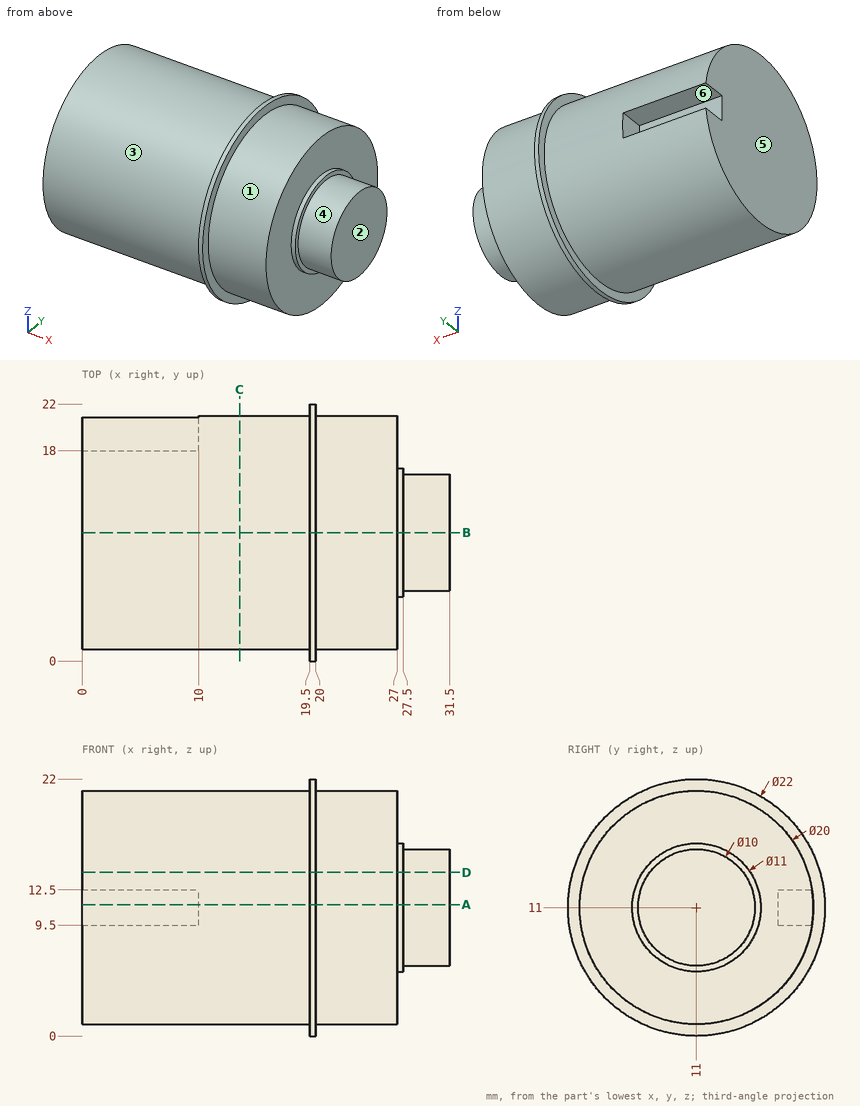
The drawing under review shows one solid part. Ordinate dimensions are in mm from its lowest x, y, z. A direction names the side the tool comes from. Round coordinates to 2 decimals unless told otherwise and drop trailing zeros. Order: outer loops, then holes, each group sorted by start corner. A loop starts at its lowest first (then second) coordinate and runs counter-clockwise, first axis right, second up. Notation, with made-up numbers: (7.25, 78.25) -> (64.25, 78.25) arc R17 cw to (64.25, 96.25) -> close; hole circle Ø5 at (65, 40.25). An arc over 180 degrees is marked (long way). Use a Markdown table: item, result.
Q1. We need section C-C on x = 13.5. Write out the cut boundary in (y, z), then the cut area to 3 significant figures.
Values:
| item | result |
|---|---|
| outline | circle Ø20 at (11, 11) |
| area | 314 mm^2 |
Q2. Clearance check with flat-ended pins moving along their axes: P1, Ø1.5, axis at y = 17.5, z = 11, coming from the +X side; P2, Ø3, axis at x = 6, y = 19.5, coming from the +Z side; P3, Ø2.5, axis at x = 6.5, y = 19.5, coming from the -Z side; P4, Ø6.5, axis at y = 12.5, z = 12.5, coming from the -X side. State where each tip first meets the part, or that it passes through.
Values:
| item | result |
|---|---|
| P1 | stops at x = 27 |
| P2 | stops at z = 18.14 |
| P3 | stops at z = 4.11 |
| P4 | stops at x = 0 |
Q3. For line 1 (X direction, y = 17.25, z = 15.25); line 2 (X direction, y = 4, z = 18.25); line 3 (Y direction, x = 29.5, z = 11.25), list the stretches that pass through material, from the lowest coordinate up.
Values:
| item | result |
|---|---|
| line 1 | x = 0 to 27 |
| line 2 | x = 19.5 to 20 |
| line 3 | y = 6.01 to 15.99 |
Q4. We need section D-D on z = 14. Write out the cut boundary in (x, y), then the cut area to 3 significant figures.
Values:
| item | result |
|---|---|
| outline | (0, 1.46) -> (19.5, 1.46) -> (19.5, 0.42) -> (20, 0.42) -> (20, 1.46) -> (27, 1.46) -> (27, 6.39) -> (27.5, 6.39) -> (27.5, 7) -> (31.5, 7) -> (31.5, 15) -> (27.5, 15) -> (27.5, 15.61) -> (27, 15.61) -> (27, 20.54) -> (20, 20.54) -> (20, 21.58) -> (19.5, 21.58) -> (19.5, 20.54) -> (0, 20.54) -> close |
| area | 553 mm^2 |
Q5. Tool access review of the marked faces 1, 2 and 3: name each direction out of +Z, -Z, +X, -X, +Y, -Y from which nothing blocks a thin tool from reaching the whole face with its end or side.
Values:
| item | result |
|---|---|
| face 1 | +X |
| face 2 | +Z, -Z, +X, +Y, -Y |
| face 3 | -X |
Q6. We need section B-B on y = 11. Write out the cut boundary in (x, z).
Values:
| item | result |
|---|---|
| outline | (0, 1) -> (19.5, 1) -> (19.5, 0) -> (20, 0) -> (20, 1) -> (27, 1) -> (27, 5.5) -> (27.5, 5.5) -> (27.5, 6) -> (31.5, 6) -> (31.5, 16) -> (27.5, 16) -> (27.5, 16.5) -> (27, 16.5) -> (27, 21) -> (20, 21) -> (20, 22) -> (19.5, 22) -> (19.5, 21) -> (0, 21) -> close |
Q7. Mouldability with a two-part tool opening along Z and no side actions: class the marked faces 4, 5 and 6 as +Z half, -Z half, draft (parallel to the pull), parting line (faces both ways), or undercut.
Values:
| item | result |
|---|---|
| face 4 | parting line |
| face 5 | draft |
| face 6 | undercut |
Q8. We need section A-A on z = 11.25. Write out the cut boundary in (x, y).
Values:
| item | result |
|---|---|
| outline | (0, 1) -> (19.5, 1) -> (19.5, 0) -> (20, 0) -> (20, 1) -> (27, 1) -> (27, 5.51) -> (27.5, 5.51) -> (27.5, 6.01) -> (31.5, 6.01) -> (31.5, 15.99) -> (27.5, 15.99) -> (27.5, 16.49) -> (27, 16.49) -> (27, 21) -> (20, 21) -> (20, 22) -> (19.5, 22) -> (19.5, 21) -> (10, 21) -> (10, 18) -> (0, 18) -> close |
